Study the drawing (mm; zero at the part's minimum x, y, z) and answer. A direction names the side the tool comes from. Give positions to 0.01 mm unless a question says otherwise; leave off trailing zeros. Loops run counter-clockwise (first coordinate to the right, second up) from the corner with the lowest first, then second, coordinate; pieces in that order, holes last. Notation, with made-up numbers: (-37.5, 43) - (3.5, 43) arc R13 ccw to (3.5, 65) - close; hole circle Ø10 at (59.25, -23.75). An arc over 180 degrees is marked (long way). Write item = value, one per line. Start each with the question number.
1) Which of the six approach directions +Z, -Z, +X, -X, +Y, -Y give full straight-line access (tool end or side, diameter ignored) to the marked faces 1, 2, 3, 4 and 5?
2) The part is cut by section A-A on y = 4.5. Write down the section's boundary in (x, z).
3) Consider probe 1 along X at (y, z) = (13.25, 13.25); probe 2 along Z at (x, y) = (4.5, 3.25); probe 3 along Z at (x, y) = (2, 13.5). Determine where each line is inside the solid, lowest interval first.
4) Flat-ended cylindrical pins translate along their axes: P1, Ø0.9, axis at x = 7, y = 2, coming from the -Z side; P2, Ø5, axis at x = 8.5, y = 3, coming from the -Z side (1 decimal); P3, Ø4.5, axis at y = 12, z = 28, coming from the -X side. Find the tip coordinate at first contact, or state that the pin passes through.
5) The mould has two halves that part along Y. Classify the marked faces 6, 7 and 8: +Y half, -Y half, draft (parallel to the pull), parting line (faces both ways), or undercut.
6) The part is cut by section B-B on z = 14.5. Write down the section's boundary in (x, y), plus the area to 3 significant figures.
7) The part is cut by section D-D on z = 2. Write down the section's boundary in (x, y), plus the area to 3 significant figures.
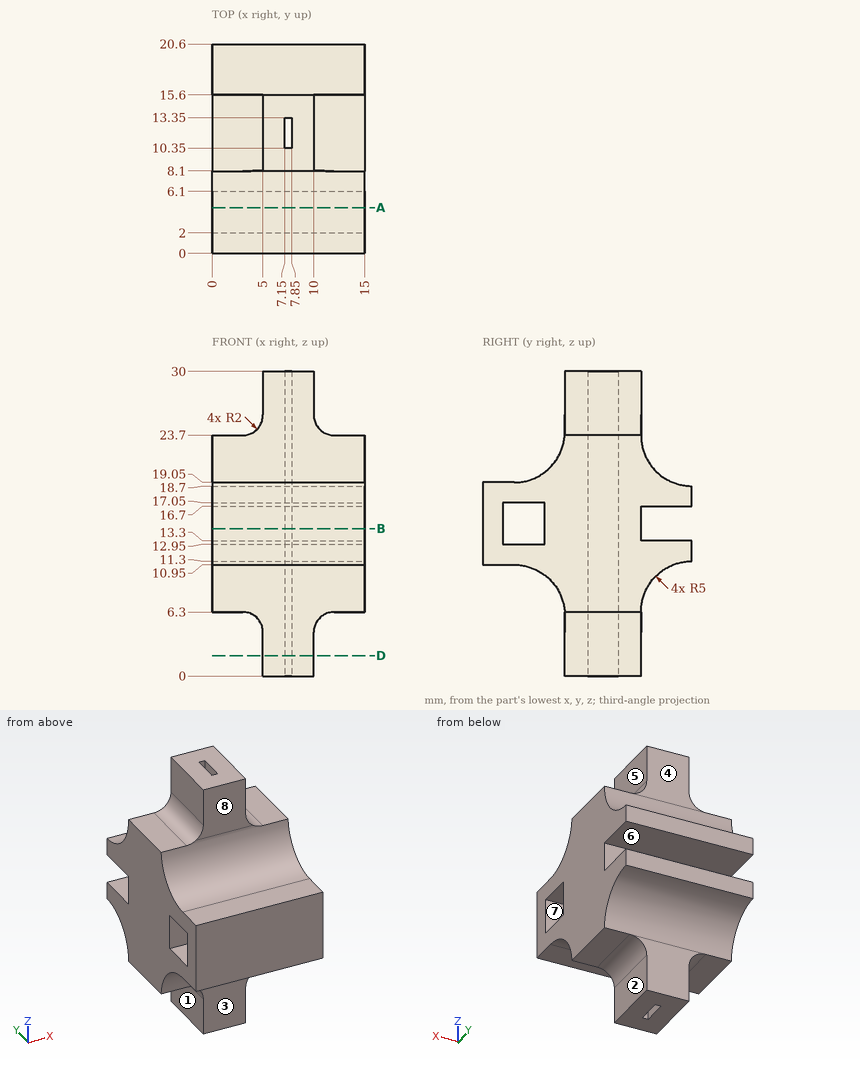
Answer below:
q1.face_1 = -Z, -X, +Y, -Y
q1.face_2 = -Z, +X, +Y, -Y
q1.face_3 = -Z, +X, -X, -Y
q1.face_4 = +Z, +X, -X, +Y
q1.face_5 = +Z, +X, +Y, -Y
q2.outline = (0, 10.75) - (15, 10.75) - (15, 12.95) - (0, 12.95) - close; (0, 17.05) - (15, 17.05) - (15, 19.25) - (0, 19.25) - close
q3.probe_1 = 0 to 7.15, 7.85 to 15
q3.probe_2 = 10.95 to 12.95, 17.05 to 19.05
q3.probe_3 = 6.3 to 23.7
q4.P1 = 10.95
q4.P2 = 10.3
q4.P3 = 5
q5.face_6 = draft
q5.face_7 = undercut
q5.face_8 = -Y half
q6.outline = (0, 0) - (15, 0) - (15, 2) - (0, 2) - close; (0, 6.1) - (15, 6.1) - (15, 15.6) - (0, 15.6) - close; hole (7.15, 10.35) - (7.85, 10.35) - (7.85, 13.35) - (7.15, 13.35) - close
q6.area = 170 mm2
q7.outline = (5, 8.1) - (10, 8.1) - (10, 15.6) - (5, 15.6) - close; hole (7.15, 10.35) - (7.85, 10.35) - (7.85, 13.35) - (7.15, 13.35) - close
q7.area = 35.4 mm2
